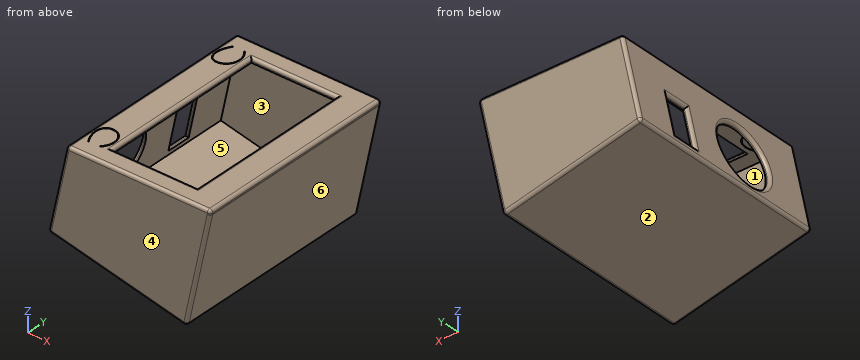
```python
from build123d import *

# Parameters (mm, degrees)
SKETCH1_W           = 48.100100719
SKETCH1_H           = 69
SKETCH1_W_2         = 45.100100719
SKETCH1_H_2         = 66
SKETCH1_W_3         = 31.49
SKETCH1_H_3         = 59.01
SKETCH1_W_4         = 28.49
SKETCH1_H_4         = 56.01
BOSS_EXTRUDE1_DEPTH = 1.5
BOSS_EXTRUDE2_REACH = 58.343
SKETCH2_W           = 47.337403978
SKETCH2_H           = 69
SKETCH2_W_2         = 44.337403978
SKETCH2_H_2         = 66
SKETCH2_3_W         = 47.337403978
SKETCH2_3_H         = 69
BOSS_EXTRUDE3_DEPTH = 1.5
CUT_EXTRUDE1_REACH  = 62.173
CUT_EXTRUDE2_REACH  = 74.28
SKETCH4_R           = 10.1542684
SKETCH4_W           = 14.182091892
SKETCH4_H           = 8.181976091
FILLET1_R           = 1


with BuildPart() as part:
    # Sketch1 → Boss-Extrude1 (new body)
    # profile 1 of 3: a face of its own
    with BuildSketch(Plane.XY):
        with Locations((-0.154741523, 0)):
            Rectangle(SKETCH1_W, SKETCH1_H)
        with Locations((-0.154741523, 0)):
            Rectangle(SKETCH1_W_2, SKETCH1_H_2, mode=Mode.SUBTRACT)
    # profile 2 of 3: a face of its own
    with BuildSketch(Plane.XY):
        with Locations((-0.154741523, 0)):
            Rectangle(SKETCH1_W_2, SKETCH1_H_2)
        Rectangle(SKETCH1_W_3, SKETCH1_H_3, mode=Mode.SUBTRACT)
    # profile 3 of 3: a face of its own
    with BuildSketch(Plane.XY):
        Rectangle(SKETCH1_W_3, SKETCH1_H_3)
        Rectangle(SKETCH1_W_4, SKETCH1_H_4, mode=Mode.SUBTRACT)
    extrude(amount=BOSS_EXTRUDE1_DEPTH)

    # Sketch2 → Boss-Extrude2 (add, up to next)
    with BuildSketch(Plane(origin=(-6.659238528, 0, -30.914212596), x_dir=(-0.9775766209565275, 0, 0.2105800326698086), z_dir=(-0.2105800326698086, 0, -0.9775766209565275)), mode=Mode.PRIVATE) as boss_extrude2_sk1:
        with Locations((0.309206719, 0)):
            Rectangle(SKETCH2_W, SKETCH2_H)
        with Locations((0.309206719, 0)):
            Rectangle(SKETCH2_W_2, SKETCH2_H_2, mode=Mode.SUBTRACT)
    boss_extrude2_tool1 = extrude(boss_extrude2_sk1.sketch, amount=-BOSS_EXTRUDE2_REACH, mode=Mode.PRIVATE) - part.part
    add(boss_extrude2_tool1.solids().sort_by_distance((-6.961512, -33.663231, -30.8491))[0])

    # Sketch2<3> → Boss-Extrude3 (add)
    with BuildSketch(Plane(origin=(-6.659238528, 0, -30.914212596), x_dir=(-0.9775766209565275, 0, 0.2105800326698086), z_dir=(-0.2105800326698086, 0, -0.9775766209565275))):
        with Locations((0.309206719, 0)):
            Rectangle(SKETCH2_3_W, SKETCH2_3_H)
    extrude(amount=BOSS_EXTRUDE3_DEPTH)

    # Sketch3 → Cut-Extrude1 (cut, up to next)
    with BuildSketch(Plane.XY.offset(1.5), mode=Mode.PRIVATE) as cut_extrude1_sk1:
        with BuildLine():
            ThreePointArc((-21.289731657, -29.000556332), (-21.318351701, -29.139051433), (-21.456846802, -29.110431389))
            add(Edge.make_bspline(
                [(-21.456846802, -29.110431389), (-21.76735388, -28.638163734), (-22.327297073, -27.617868396), (-23.022339766, -25.632974806), (-23.184429728, -23.286569664), (-22.349812004, -21.534860233), (-21.046397057, -20.801758586), (-19.804512561, -20.676612388), (-18.519292443, -20.934519944), (-17.050207703, -21.781257639), (-16.078766807, -23.226153574), (-15.74627905, -24.98133739), (-15.854990247, -26.382669418), (-16.279006649, -27.565007319), (-16.828982995, -28.475116006), (-17.189531054, -28.926049006), (-17.379130961, -29.134965143)],
                knots=[0, 0, 0, 0, 0.0625, 0.125, 0.25, 0.375, 0.4375, 0.5, 0.5625, 0.625, 0.75, 0.8125, 0.875, 0.9375, 0.96875, 1, 1, 1, 1], degree=3))
            ThreePointArc((-17.379130961, -29.134965143), (-17.520386483, -29.141811854), (-17.527233194, -29.000556332))
            add(Edge.make_bspline(
                [(-21.289731657, -29.000556332), (-23.500889651, -25.637481941), (-23.314330036, -20.653187448), (-16.260242518, -21.102744912), (-14.890038838, -26.094687506), (-17.527233194, -29.000556332)],
                knots=[0, 0, 0, 0, 0.438563054, 0.566022066, 1, 1, 1, 1], degree=3))
        make_face()
    cut_extrude1_tool1 = extrude(cut_extrude1_sk1.sketch, amount=-CUT_EXTRUDE1_REACH, mode=Mode.PRIVATE) & part.part
    # Sketch3 → Cut-Extrude1 (cut, up to next)
    with BuildSketch(Plane.XY.offset(1.5), mode=Mode.PRIVATE) as cut_extrude1_sk2:
        with BuildLine():
            add(Edge.make_bspline(
                [(-21.456846802, 29.110431389), (-21.76735388, 28.638163734), (-22.327297073, 27.617868396), (-23.022339766, 25.632974806), (-23.184429728, 23.286569664), (-22.349812004, 21.534860233), (-21.046397057, 20.801758586), (-19.804512561, 20.676612388), (-18.519292443, 20.934519944), (-17.050207703, 21.781257639), (-16.078766807, 23.226153574), (-15.74627905, 24.98133739), (-15.854990247, 26.382669418), (-16.279006649, 27.565007319), (-16.828982995, 28.475116006), (-17.189531054, 28.926049006), (-17.379130961, 29.134965143)],
                knots=[0, 0, 0, 0, 0.0625, 0.125, 0.25, 0.375, 0.4375, 0.5, 0.5625, 0.625, 0.75, 0.8125, 0.875, 0.9375, 0.96875, 1, 1, 1, 1], degree=3))
            ThreePointArc((-17.379130961, 29.134965143), (-17.520386483, 29.141811854), (-17.527233194, 29.000556332))
            add(Edge.make_bspline(
                [(-21.289731657, 29.000556332), (-23.500889651, 25.637481941), (-23.314330036, 20.653187448), (-16.260242518, 21.102744912), (-14.890038838, 26.094687506), (-17.527233194, 29.000556332)],
                knots=[0, 0, 0, 0, 0.438563054, 0.566022066, 1, 1, 1, 1], degree=3))
            ThreePointArc((-21.289731657, 29.000556332), (-21.318351701, 29.139051433), (-21.456846802, 29.110431389))
        make_face()
    cut_extrude1_tool2 = extrude(cut_extrude1_sk2.sketch, amount=-CUT_EXTRUDE1_REACH, mode=Mode.PRIVATE) & part.part
    add(cut_extrude1_tool1.solids().sort_by_distance((-21.379464, -29.046102, 1.5))[0], mode=Mode.SUBTRACT)
    add(cut_extrude1_tool2.solids().sort_by_distance((-19.655611, 20.861949, 1.5))[0], mode=Mode.SUBTRACT)

    # Sketch4 → Cut-Extrude2 (cut, up to next)
    with BuildSketch(Plane(origin=(-23.440242972, 0, 5.049268799), x_dir=(0.21058003266980863, 0, 0.9775766209565275), z_dir=(-0.9775766209565275, 0, 0.21058003266980863)), mode=Mode.PRIVATE) as cut_extrude2_sk1:
        with Locations((-20.323314156, -10.4)):
            Circle(SKETCH4_R)
    cut_extrude2_tool1 = extrude(cut_extrude2_sk1.sketch, amount=-CUT_EXTRUDE2_REACH, mode=Mode.PRIVATE) & part.part
    # Sketch4 → Cut-Extrude2 (cut, up to next)
    with BuildSketch(Plane(origin=(-23.440242972, 0, 5.049268799), x_dir=(0.21058003266980863, 0, 0.9775766209565275), z_dir=(-0.9775766209565275, 0, 0.21058003266980863)), mode=Mode.PRIVATE) as cut_extrude2_sk2:
        with Locations((-22.959694985, 15.523026861)):
            Rectangle(SKETCH4_W, SKETCH4_H)
    cut_extrude2_tool2 = extrude(cut_extrude2_sk2.sketch, amount=-CUT_EXTRUDE2_REACH, mode=Mode.PRIVATE) & part.part
    add(cut_extrude2_tool1.solids().sort_by_distance((-27.719927, -10.4, -14.818328))[0], mode=Mode.SUBTRACT)
    add(cut_extrude2_tool2.solids().sort_by_distance((-28.275096, 15.523027, -17.395592))[0], mode=Mode.SUBTRACT)

    # Fillet1
    fillet1_edges = [part.edges().sort_by_distance(p)[0] for p in [
        (23.895308837, 0, 0),
        (-29.858213302, -10.4, -24.744903371),
        (-29.768328979, 15.523026862, -24.327632977),
        (-28.275096292, 11.432038816, -17.395592243),
        (-26.781863605, 15.523026862, -10.463551508),
        (-28.275096292, 19.614014907, -17.395592243),
        (0, 28.005, 1.5),
        (14.245, 0, 1.5),
        (23.895308837, 34.5, 0.75),
        (23.895308837, -34.5, 0.75),
        (0, -28.005, 1.5),
        (-0.154741522, 34.5, 1.5),
        (-27.310071715, 34.5, -12.915654364),
        (-24.204791882, 0, 1.5),
        (19.877948357, 34.5, -18.649810402),
        (-27.310071715, -34.5, -12.915654364),
        (19.877948357, -34.5, -18.649810402),
        (-0.154741522, -34.5, 1.5),
        (23.895308837, 0, 1.5),
        (15.860587876, 0, -37.299620805),
        (-7.277381836, 34.5, -32.315464767),
        (-7.277381836, -34.5, -32.315464767),
        (-30.415351549, 0, -27.331308728),
        (-14.245, 0, 1.5),
    ]]
    fillet(fillet1_edges, radius=FILLET1_R)


solid = part.part
```
Can you work these out from the model? Positions are in its coordinate system, mm. Face numbers are marked on the shaded views. A direction names the side the tool comes from. Coordinates: 2 decimals unless noted, no trailing zeros. Use a Markdown table: item, result.
Item 1: I want a section at B-B on y = -26. Give the number of separate pieces and of enclosed holes in the cut face, and give its area (3 significant figures).
Numbers:
| item | result |
|---|---|
| separate pieces | 3 |
| enclosed holes | 0 |
| area | 194 mm2 |
Item 2: Will these pins go through, and if not, where does the flat tip stop? pin 1 (4 mm diameter, centred on x = -7.5, y = 0, fed in from -Z); pin 2 (1.5 mm diameter, centred on y = 20.5, z = -16, fed in from +X); pin 3 (8 mm diameter, centred on y = 8.5, z = -7, fed in from -X).
Numbers:
| item | result |
|---|---|
| pin 1 | stops at z = -32.7 |
| pin 2 | stops at x = 20.61 |
| pin 3 | stops at x = -26.9 |
Item 3: For the marked faces 5 and 6, which set-ups out of +Z, -Z, +X, -X, +Y, -Y let a thin tool reach every point of the face, with its end or its side?
Numbers:
| item | result |
|---|---|
| face 5 | none |
| face 6 | -Z, +X, +Y, -Y |
Item 4: We'd pull the mould along Y, two halves only. Please class the marked faces 1, 2, 3 and 4: released by +Y, released by -Y, zero draft, split by the parting line, or undercut.
Numbers:
| item | result |
|---|---|
| face 1 | undercut |
| face 2 | zero draft |
| face 3 | undercut |
| face 4 | released by -Y |
Item 5: If I drill on probe 1 along Y at (x, z) = (-16.5, -2.5); probe 2 along Z at (x, y) = (-15, 24.5); probe 3 along X at (y, z) = (22, -20), over which ranges is the centre line in solid material (lowest first)? Write a range as from..to.
Numbers:
| item | result |
|---|---|
| probe 1 | y = -34.5..-33, 33..34.5 |
| probe 2 | z = -30.65..-29.12, 0..1.47 |
| probe 3 | x = -28.84..-27.3, 18.05..19.59 |
